```python
from build123d import *

# Parameters (mm, degrees)
BOSS_EXTRUDE1_DEPTH                 = 22.225
FILLET1_R                           = 3.175
FILLET2_R                           = 25.4
SKETCH3_R                           = 7.14375
CUT_EXTRUDE1_DEPTH                  = 9.525
SKETCH4_R                           = 4.25
CUT_EXTRUDE2_DEPTH                  = 58.15
F_7_32_0_21875_DIAMETER_HOLE1_D     = 5.55625
F_7_32_0_21875_DIAMETER_HOLE1_DEPTH = 7.9375
F_7_32_0_21875_DIAMETER_HOLE1_TIP   = 1.669265907
SKETCH9_R                           = 1.984375
CUT_EXTRUDE3_DEPTH                  = 23.2250001
SKETCH10_R                          = 1.984375
CUT_EXTRUDE4_DEPTH                  = 23.2250001


with BuildPart() as part:
    # Sketch1 → Boss-Extrude1 (new body)
    with BuildSketch(Plane.XY):
        Polygon((0, 0), (0, 57.15), (38.1, 57.15), (38.1, 19.05), (22.225, 19.05), (22.225, 0), align=None)
    extrude(amount=BOSS_EXTRUDE1_DEPTH)

    # Fillet1
    fillet1_edges = [part.edges().sort_by_distance(p)[0] for p in [
        (22.225, 19.05, 11.1125),
    ]]
    fillet(fillet1_edges, radius=FILLET1_R)

    # Fillet2
    fillet2_edges = [part.edges().sort_by_distance(p)[0] for p in [
        (0, 57.15, 11.1125),
    ]]
    fillet(fillet2_edges, radius=FILLET2_R)

    # Sketch3 → Cut-Extrude1 (cut)
    with BuildSketch(Plane.XZ):
        with Locations((11.1125, 11.1125)):
            Circle(SKETCH3_R)
    extrude(amount=-CUT_EXTRUDE1_DEPTH, mode=Mode.SUBTRACT)

    # Sketch4 → Cut-Extrude2 (cut, through all)
    with BuildSketch(Plane.XZ):
        with Locations((11.1125, 11.1125)):
            Circle(SKETCH4_R)
    extrude(amount=-CUT_EXTRUDE2_DEPTH, mode=Mode.SUBTRACT)

    # 7/32 (0.21875) Diameter Hole1
    with Locations(Plane(origin=(38.1, 0, 0), x_dir=(0, 0, -1), z_dir=(1, 0, 0))):
        with Locations((-11.1125, 50.8), (-11.1125, 25.4)):
            Hole(F_7_32_0_21875_DIAMETER_HOLE1_D / 2, depth=F_7_32_0_21875_DIAMETER_HOLE1_DEPTH)
            with Locations((0, 0, -(F_7_32_0_21875_DIAMETER_HOLE1_DEPTH + F_7_32_0_21875_DIAMETER_HOLE1_TIP / 2))):  # 118° drill point
                Cone(0, F_7_32_0_21875_DIAMETER_HOLE1_D / 2, F_7_32_0_21875_DIAMETER_HOLE1_TIP, mode=Mode.SUBTRACT)

    # Sketch9 → Cut-Extrude3 (cut, through all)
    with BuildSketch(Plane(origin=(22.225, 0, 0), x_dir=(0, 0, -1), z_dir=(1, 0, 0))):
        with Locations((-11.1125, 12.7)):
            Circle(SKETCH9_R)
    extrude(amount=-CUT_EXTRUDE3_DEPTH, mode=Mode.SUBTRACT)

    # Sketch10 → Cut-Extrude4 (cut, through all)
    with BuildSketch(Plane.XY.offset(22.225)):
        with Locations((11.1125, 12.7)):
            Circle(SKETCH10_R)
    extrude(amount=-CUT_EXTRUDE4_DEPTH, mode=Mode.SUBTRACT)


solid = part.part
```
Input: part model. Units: mm. Frame: model coordinates. A direction names the side the tool comes from. Round coordinates to 2 decimals unless told otherwise and drop trailing zeros. Loops run counter-clockwise (first coordinate to the right, second up) from the corner with the lowest first, then second, coordinate; pieces in that order, holes last. Notation, with made-up numbers: (74.25, 21) -> (127.25, 21) arc R8 cw to (127.25, 26) -> close; hole circle Ø9 at (10.5, 18). An arc over 180 degrees is marked (long way). Write each question's results on one line, items separated by ' | '.
1. Section D-D (x = 10.5). Return loops of the section in (y, z) (3 decimals), and give its area (3 significant figures).
Geometry results:
outline: (0, 0) -> (10.813, 0) -> (10.813, 6.907) -> (9.525, 6.907) -> (9.525, 3.995) -> (0, 3.995) -> close; (0, 18.23) -> (9.525, 18.23) -> (9.525, 15.318) -> (10.813, 15.318) -> (10.813, 22.225) -> (0, 22.225) -> close; (14.587, 0) -> (52.321, 0) -> (52.321, 6.907) -> (14.587, 6.907) -> close; (14.587, 15.318) -> (52.321, 15.318) -> (52.321, 22.225) -> (14.587, 22.225) -> close | area: 615 mm2
2. Mould query, pull axis Z, two halves, no side actions, for faces 5 (the face through (23.18, 18.145, 11.268)), 6 (the face through (11, 9.525, 6)), 7 (the face through (28.783, 50.506, 11.495)), 8 (the face through (19, 29, 0)). Classes: +Z half, -Z half, draft (parallel to the pull), parting line (faces both ways), or undercut.
Geometry results:
face 5: draft | face 6: undercut | face 7: undercut | face 8: -Z half
3. First-contact query: P1, Ø11.5, axis at x = 13.5, z = 12, coming from the -Y side; P2, Ø10, axis at x = 11.11, z = 11.11, coming from the +Y side; P3, Ø13, axis at x = 11.11, z = 11.11, coming from the +Y side; P4, Ø4.5, axis at y = 50.8, z = 11.11, coming from the -X side. Flat tips, straight axial feed; report the tip coordinate or a pass-through.
Geometry results:
P1: y = 0 | P2: y = 55.39 | P3: y = 55.93 | P4: x = 6.35
4. Section B-B (y = 12.7). State how many separate pieces and enclosed holes the cut face has, and give its area (3 significant figures).
Geometry results:
separate pieces: 4 | enclosed holes: 0 | area: 326 mm2
5. Ray query, line 1 (X direction, y = 12.7, z = 17.5) (3 decimals); line 2 (Z direction, x = 33.5, y = 25.4) (3 decimals). Return the intervals inside material, ascending. Write a range as from..to.
Geometry results:
line 1: 0..9.128, 13.097..22.225 | line 2: 0..8.334, 13.891..22.225
6. Set-up query: faces 1 (the face through (22.225, 8, 11)), 2 (the face through (0, 16, 11)), 3 (the face through (10.183, 4.696, 18.195)), 4 (the face through (34.076, 28.154, 10.751)). Return all of +Z, -Z, +X, -X, +Y, -Y with unobstructed straight access to the full face (end or side cutting, diameter ignored); none if empty.
Geometry results:
face 1: +Z, -Z, +X, -Y | face 2: +Z, -Z, -X, +Y, -Y | face 3: -Y | face 4: +X
